Can you work these out from the model? Positions are in its coordinate system, mm. A direction names the side the tool comes from. Round coordinates to 2 decimals unless told otherwise and drop trailing zeros. Order: outer loops, then holes, each group sorted by start corner. A loop starts at its lowest first (then second) coordinate and runs counter-clockwise, first axis right, second up. Notation, with made-up numbers: (8.25, 42) -> (55.25, 42) arc R25 cw to (55.25, 62) -> close; hole circle Ø5 at (-25, -21.75). An arc over 180 degrees is marked (long way). One line per item, written item: value.
```python
from build123d import *

# Parameters (mm, degrees)
BOSS_EXTRUDE2_DEPTH = 20
SKETCH1_3_R         = 10
SKETCH1_3_R_2       = 5
BOSS_EXTRUDE3_DEPTH = 3
SHELL1_DEPTH        = 18
SHELL1_2_OUTLINE_R  = 5
SHELL1_2_DEPTH      = 1


# Read off the part's stored shape, not the designer's step: Shell1
with BuildPart() as part:
    # Sketch1 → Boss-Extrude2 (new body)
    with BuildSketch(Plane.XY):
        with BuildLine():
            ThreePointArc((-40, 0), (-42.583801513, -6.708203932), (-49, -9.949874371))
            ThreePointArc((-49, -9.949874371), (-43.301270189, -25), (-33.11684397, -37.4603076))
            ThreePointArc((-33.11684397, -37.4603076), (-21.931485677, -33.783695926), (-15, -43.301270189))
            ThreePointArc((-15, -43.301270189), (-15.223281744, -45.402645965), (-15.88315603, -47.410181971))
            ThreePointArc((-15.88315603, -47.410181971), (0, -50), (15.88315603, -47.410181971))
            ThreePointArc((15.88315603, -47.410181971), (20, -34.641016151), (33.11684397, -37.4603076))
            ThreePointArc((33.11684397, -37.4603076), (43.301270189, -25), (49, -9.949874371))
            ThreePointArc((49, -9.949874371), (40, 0), (49, 9.949874371))
            ThreePointArc((49, 9.949874371), (43.301270189, 25), (33.11684397, 37.4603076))
            ThreePointArc((33.11684397, 37.4603076), (20, 34.641016151), (15.88315603, 47.410181971))
            ThreePointArc((15.88315603, 47.410181971), (0, 50), (-15.88315603, 47.410181971))
            ThreePointArc((-15.88315603, 47.410181971), (-15.223281744, 45.402645965), (-15, 43.301270189))
            ThreePointArc((-15, 43.301270189), (-21.931485677, 33.783695926), (-33.11684397, 37.4603076))
            ThreePointArc((-33.11684397, 37.4603076), (-43.301270189, 25), (-49, 9.949874371))
            ThreePointArc((-49, 9.949874371), (-42.583801513, 6.708203932), (-40, 0))
        make_face()
        with BuildLine():
            ThreePointArc((24.748737342, -24.748737342), (13.393920133, -32.335783638), (0, -35))
            ThreePointArc((0, -35), (-5, -30), (0, -25))
            ThreePointArc((0, -25), (9.567085809, -23.096988313), (17.67766953, -17.67766953))
            ThreePointArc((17.67766953, -17.67766953), (24.748737342, -17.67766953), (24.748737342, -24.748737342))
        make_face(mode=Mode.SUBTRACT)
        with BuildLine():
            ThreePointArc((-33.80740392, -9.058666579), (-34.700570148, 4.568416728), (-30.310889132, 17.5))
            ThreePointArc((-30.310889132, 17.5), (-23.480762114, 19.330127019), (-21.650635095, 12.5))
            ThreePointArc((-21.650635095, 12.5), (-24.786121534, 3.263154806), (-24.148145657, -6.470476128))
            ThreePointArc((-24.148145657, -6.470476128), (-27.683679563, -12.594200485), (-33.80740392, -9.058666579))
        make_face(mode=Mode.SUBTRACT)
        with BuildLine():
            ThreePointArc((9.058666579, 33.80740392), (21.306650015, 27.76736691), (30.310889132, 17.5))
            ThreePointArc((30.310889132, 17.5), (28.480762114, 10.669872981), (21.650635095, 12.5))
            ThreePointArc((21.650635095, 12.5), (15.219035725, 19.833833507), (6.470476128, 24.148145657))
            ThreePointArc((6.470476128, 24.148145657), (2.934942222, 30.271870014), (9.058666579, 33.80740392))
        make_face(mode=Mode.SUBTRACT)
    extrude(amount=BOSS_EXTRUDE2_DEPTH)

    # Sketch1<3> → Boss-Extrude3 (add)
    # profile 1 of 6: a face of its own
    with BuildSketch(Plane.XY):
        with Locations((50, 0)):
            Circle(SKETCH1_3_R)
        with Locations((50, 0)):
            Circle(SKETCH1_3_R_2, mode=Mode.SUBTRACT)
    # profile 2 of 6: a face of its own
    with BuildSketch(Plane.XY):
        with Locations((25, -43.301270189)):
            Circle(SKETCH1_3_R)
        with Locations((25, -43.301270189)):
            Circle(SKETCH1_3_R_2, mode=Mode.SUBTRACT)
    # profile 3 of 6: a face of its own
    with BuildSketch(Plane.XY):
        with Locations((-25, -43.301270189)):
            Circle(SKETCH1_3_R)
        with Locations((-25, -43.301270189)):
            Circle(SKETCH1_3_R_2, mode=Mode.SUBTRACT)
    # profile 4 of 6: a face of its own
    with BuildSketch(Plane.XY):
        with Locations((-50, 0)):
            Circle(SKETCH1_3_R)
        with Locations((-50, 0)):
            Circle(SKETCH1_3_R_2, mode=Mode.SUBTRACT)
    # profile 5 of 6: a face of its own
    with BuildSketch(Plane.XY):
        with Locations((-25, 43.301270189)):
            Circle(SKETCH1_3_R)
        with Locations((-25, 43.301270189)):
            Circle(SKETCH1_3_R_2, mode=Mode.SUBTRACT)
    # profile 6 of 6: a face of its own
    with BuildSketch(Plane.XY):
        with Locations((25, 43.301270189)):
            Circle(SKETCH1_3_R)
        with Locations((25, 43.301270189)):
            Circle(SKETCH1_3_R_2, mode=Mode.SUBTRACT)
    extrude(amount=BOSS_EXTRUDE3_DEPTH)

    # Shell1 outline → Shell1 (cut)
    with BuildSketch(Plane.XY):
        with BuildLine():
            ThreePointArc((46.6, 11.508257905), (41.569219382, 24), (33.266443699, 34.602654864))
            ThreePointArc((33.266443699, 34.602654864), (19, 32.908965344), (13.333556301, 46.110912769))
            ThreePointArc((13.333556301, 46.110912769), (0, 48), (-13.333556301, 46.110912769))
            ThreePointArc((-13.333556301, 46.110912769), (-19, 32.908965344), (-33.266443699, 34.602654864))
            ThreePointArc((-33.266443699, 34.602654864), (-41.569219382, 24), (-46.6, 11.508257905))
            ThreePointArc((-46.6, 11.508257905), (-38, 0), (-46.6, -11.508257905))
            ThreePointArc((-46.6, -11.508257905), (-41.569219382, -24), (-33.266443699, -34.602654864))
            ThreePointArc((-33.266443699, -34.602654864), (-19, -32.908965344), (-13.333556301, -46.110912769))
            ThreePointArc((-13.333556301, -46.110912769), (0, -48), (13.333556301, -46.110912769))
            ThreePointArc((13.333556301, -46.110912769), (19, -32.908965344), (33.266443699, -34.602654864))
            ThreePointArc((33.266443699, -34.602654864), (41.569219382, -24), (46.6, -11.508257905))
            ThreePointArc((46.6, -11.508257905), (38, 0), (46.6, 11.508257905))
        make_face()
        with BuildLine():
            ThreePointArc((17.67766953, -17.67766953), (24.748737342, -17.67766953), (24.748737342, -24.748737342))
            ThreePointArc((24.748737342, -24.748737342), (13.393920133, -32.335783638), (0, -35))
            ThreePointArc((0, -35), (-5, -30), (0, -25))
            ThreePointArc((0, -25), (9.567085809, -23.096988313), (17.67766953, -17.67766953))
        make_face(mode=Mode.SUBTRACT)
        with BuildLine():
            ThreePointArc((-21.650635095, 12.5), (-24.786121534, 3.263154805), (-24.148145657, -6.470476128))
            ThreePointArc((-24.148145657, -6.470476128), (-27.683679563, -12.594200485), (-33.80740392, -9.058666579))
            ThreePointArc((-33.80740392, -9.058666579), (-34.700570148, 4.568416728), (-30.310889132, 17.5))
            ThreePointArc((-30.310889132, 17.5), (-23.480762113, 19.330127019), (-21.650635095, 12.5))
        make_face(mode=Mode.SUBTRACT)
        with BuildLine():
            ThreePointArc((6.470476128, 24.148145657), (2.934942222, 30.271870014), (9.058666579, 33.80740392))
            ThreePointArc((9.058666579, 33.80740392), (21.306650015, 27.76736691), (30.310889132, 17.5))
            ThreePointArc((30.310889132, 17.5), (28.480762114, 10.669872981), (21.650635095, 12.5))
            ThreePointArc((21.650635095, 12.5), (15.219035725, 19.833833507), (6.470476128, 24.148145657))
        make_face(mode=Mode.SUBTRACT)
    extrude(amount=SHELL1_DEPTH, mode=Mode.SUBTRACT)

    # Shell1 2 outline → Shell1 2 (cut)
    # profile 1 of 6: a face of its own
    with BuildSketch(Plane.XY):
        with BuildLine():
            ThreePointArc((13.333556301, 46.110912769), (19, 32.908965344), (33.266443699, 34.602654864))
            ThreePointArc((33.266443699, 34.602654864), (31.787193359, 35.966294477), (30.2520989, 37.266748076))
            ThreePointArc((30.2520989, 37.266748076), (29, 50.229473419), (17.1479011, 44.832460203))
            ThreePointArc((17.1479011, 44.832460203), (15.254128017, 45.511664202), (13.333556301, 46.110912769))
        make_face()
        with Locations((25, 43.301270189)):
            Circle(SHELL1_2_OUTLINE_R, mode=Mode.SUBTRACT)
    # profile 2 of 6: a face of its own
    with BuildSketch(Plane.XY):
        with BuildLine():
            ThreePointArc((47.4, 7.565712128), (47.041321376, 9.545369726), (46.6, 11.508257905))
            ThreePointArc((46.6, 11.508257905), (38, 0), (46.6, -11.508257905))
            ThreePointArc((46.6, -11.508257905), (47.041321376, -9.545369726), (47.4, -7.565712128))
            ThreePointArc((47.4, -7.565712128), (58, 0), (47.4, 7.565712128))
        make_face()
        with Locations((50, 0)):
            Circle(SHELL1_2_OUTLINE_R, mode=Mode.SUBTRACT)
    # profile 3 of 6: a face of its own
    with BuildSketch(Plane.XY):
        with BuildLine():
            ThreePointArc((-33.266443699, 34.602654864), (-19, 32.908965344), (-13.333556301, 46.110912769))
            ThreePointArc((-13.333556301, 46.110912769), (-15.254128017, 45.511664202), (-17.1479011, 44.832460203))
            ThreePointArc((-17.1479011, 44.832460203), (-29, 50.229473419), (-30.2520989, 37.266748076))
            ThreePointArc((-30.2520989, 37.266748076), (-31.787193359, 35.966294477), (-33.266443699, 34.602654864))
        make_face()
        with Locations((-25, 43.301270189)):
            Circle(SHELL1_2_OUTLINE_R, mode=Mode.SUBTRACT)
    # profile 4 of 6: a face of its own
    with BuildSketch(Plane.XY):
        with BuildLine():
            ThreePointArc((30.2520989, -37.266748076), (31.787193359, -35.966294477), (33.266443699, -34.602654864))
            ThreePointArc((33.266443699, -34.602654864), (19, -32.908965344), (13.333556301, -46.110912769))
            ThreePointArc((13.333556301, -46.110912769), (15.254128017, -45.511664202), (17.1479011, -44.832460203))
            ThreePointArc((17.1479011, -44.832460203), (29, -50.229473419), (30.2520989, -37.266748076))
        make_face()
        with Locations((25, -43.301270189)):
            Circle(SHELL1_2_OUTLINE_R, mode=Mode.SUBTRACT)
    # profile 5 of 6: a face of its own
    with BuildSketch(Plane.XY):
        with BuildLine():
            ThreePointArc((-46.6, -11.508257905), (-38, 0), (-46.6, 11.508257905))
            ThreePointArc((-46.6, 11.508257905), (-47.041321376, 9.545369726), (-47.4, 7.565712128))
            ThreePointArc((-47.4, 7.565712128), (-58, 0), (-47.4, -7.565712128))
            ThreePointArc((-47.4, -7.565712128), (-47.041321376, -9.545369726), (-46.6, -11.508257905))
        make_face()
        with Locations((-50, 0)):
            Circle(SHELL1_2_OUTLINE_R, mode=Mode.SUBTRACT)
    # profile 6 of 6: a face of its own
    with BuildSketch(Plane.XY):
        with BuildLine():
            ThreePointArc((-17.1479011, -44.832460203), (-15.254128017, -45.511664202), (-13.333556301, -46.110912769))
            ThreePointArc((-13.333556301, -46.110912769), (-19, -32.908965344), (-33.266443699, -34.602654864))
            ThreePointArc((-33.266443699, -34.602654864), (-31.787193359, -35.966294477), (-30.2520989, -37.266748076))
            ThreePointArc((-30.2520989, -37.266748076), (-29, -50.229473419), (-17.1479011, -44.832460203))
        make_face()
        with Locations((-25, -43.301270189)):
            Circle(SHELL1_2_OUTLINE_R, mode=Mode.SUBTRACT)
    extrude(amount=SHELL1_2_DEPTH, mode=Mode.SUBTRACT)


solid = part.part
```
Q1. I want a section at C-C on x = -8.5. List the corners of the cut face in (y, z) for me, plus the area to 3 significant figures.
Answers below:
outline: (-49.27, 0) -> (-47.24, 0) -> (-47.24, 18) -> (47.24, 18) -> (47.24, 0) -> (49.27, 0) -> (49.27, 20) -> (-49.27, 20) -> close
area: 270 mm^2
Q2. I want a section at A-A on z = 12.75. List the corners of the cut face in (x, y) for me.
Answers below:
outline: (-49, -9.95) arc R50 ccw to (-33.12, -37.46) arc R10 cw to (-15.88, -47.41) arc R50 ccw to (15.88, -47.41) arc R10 cw to (33.12, -37.46) arc R50 ccw to (49, -9.95) arc R10 cw to (49, 9.95) arc R50 ccw to (33.12, 37.46) arc R10 cw to (15.88, 47.41) arc R50 ccw to (-15.88, 47.41) arc R10 cw to (-33.12, 37.46) arc R50 ccw to (-49, 9.95) arc R10 cw to start; hole (-46.6, -11.51) arc R48 ccw to (-33.27, -34.6) arc R12 cw to (-13.33, -46.11) arc R48 ccw to (13.33, -46.11) arc R12 cw to (33.27, -34.6) arc R48 ccw to (46.6, -11.51) arc R12 cw to (46.6, 11.51) arc R48 ccw to (33.27, 34.6) arc R12 cw to (13.33, 46.11) arc R48 ccw to (-13.33, 46.11) arc R12 cw to (-33.27, 34.6) arc R48 ccw to (-46.6, 11.51) arc R12 cw to start
Q3. Will these pins go through, and if not, where does the flat tip stop? pin 1 Ø1.5 at (x, y) = (-36, -10.5) entering from -Z; pin 2 Ø6 at (x, y) = (23, 38) entering from -Z; pin 3 Ø1.5 at (x, z) = (40, 12.5) entering from -Y; pin 4 Ø10 at (x, y) = (52.5, 3) entering from -Z.
Answers below:
pin 1: z = 18
pin 2: z = 1
pin 3: y = -30.97
pin 4: z = 0
Q4. Please list where these lines run through material, in increasing order: line 1 along Y through (x, z) = (50, 2.5); line 2 along Y through (x, z) = (-50, 0.6); line 3 along X through (y, z) = (0, 0.6).
Answers below:
line 1: -10 to -5, 5 to 10
line 2: -10 to -8, 8 to 10
line 3: -60 to -58, 58 to 60
Q5. On a 3-axis mill with a long thin cutter (end or side, diameter ignored), from which of +Z, -Z, +X, -X, +Y, -Y can I reach the whole of each face in a straight line? I mean faces 1 (the face through (28.814, -50.334, 0.493)), 2 (the face through (-24.768, 3.399, 18.986)). Say none if no direction works.
Answers below:
face 1: -Z
face 2: +Z, -Z
Q6. I want a section at B-B on y = -30. List the corners of the cut face in (x, z) for me.
Answers below:
outline: (-40, 0) -> (-37.47, 0) -> (-37.47, 18) -> (-5, 18) -> (-5, 20) -> (-40, 20) -> close; (18.03, 18) -> (37.47, 18) -> (37.47, 0) -> (40, 0) -> (40, 20) -> (18.03, 20) -> close
Q7. We'd pull the mould along Y, two halves only. Please class faces 3 (the face through (60, 0, 1)), 4 (the face through (29.183, 50.121, 0.493)): released by +Y, released by -Y, zero draft, split by the parting line, or undercut.
Answers below:
face 3: split by the parting line
face 4: undercut
